For this review, take the finished solid that the model builds, in its own axes (mm). Face numbers are marked on the shaded views. Coordinates: 2 decimals unless noted, no trailing zeros. Order: outer loops, then holes, each group sorted by start corner. A loop starts at its lowest first (then second) coordinate and runs counter-clockwise, first axis right, second up. Notation, with made-up numbers: M 72,27 L 128,27 A29 ccw 128,61 Z; hole C 68.25,-2 d5. An arc over 180 degrees is marked long. Use CSV: the item, a comma, the result in double quotes.
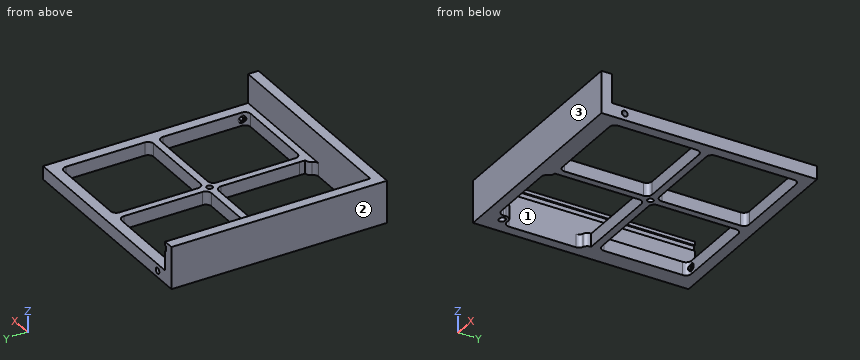
```python
from build123d import *

# Parameters (mm, degrees)
BOSS_EXTRUDE1_DEPTH            = 23
SKETCH2_W                      = 3
SKETCH2_H                      = 112
CUT_EXTRUDE1_DEPTH             = 0.75
SKETCH3_W                      = 7.2
SKETCH3_H                      = 6
BOSS_EXTRUDE2_DEPTH            = 10
SKETCH3_3_W                    = 7.2
SKETCH3_3_H                    = 106
BOSS_EXTRUDE3_DEPTH            = 4
FILLET1_R                      = 3
SKETCH5_W                      = 101.3
SKETCH5_H                      = 7.2
BOSS_EXTRUDE4_DEPTH            = 4
SKETCH5_3_W                    = 6
SKETCH5_3_H                    = 7.2
BOSS_EXTRUDE5_DEPTH            = 10
FILLET3_R                      = 3
SKETCH6_W                      = 50
SKETCH6_H                      = 50
CUT_EXTRUDE2_DEPTH             = 167.709117927
FILLET8_R                      = 3
FILLET9_R                      = 3
FILLET10_R                     = 3
FILLET11_R                     = 3
CUT_EXTRUDE3_REACH             = 169.545
SKETCH7_R                      = 1
CUT_EXTRUDE3_DIRECTION_2_DEPTH = 168.544889647
SKETCH7_5_R                    = 1.6
SKETCH7_5_R_2                  = 1
CUT_EXTRUDE4_DEPTH             = 3.2
CUT_EXTRUDE6_START             = -5.5
SKETCH8_R                      = 2
CUT_EXTRUDE6_DEPTH             = 3
CUT_EXTRUDE7_REACH             = 169.545
SKETCH9_R                      = 1
SKETCH9_3_R                    = 1.6
SKETCH9_3_R_2                  = 1
CUT_EXTRUDE8_DEPTH             = 3.2
CUT_EXTRUDE9_START             = -5.5
SKETCH10_R                     = 2
CUT_EXTRUDE9_DEPTH             = 3.2
BOSS_EXTRUDE6_DEPTH            = 7.2
FILLET12_R                     = 3
BOSS_EXTRUDE7_DEPTH            = 7.2
FILLET13_R                     = 3
FILLET14_R                     = 3
FILLET15_R                     = 3
FILLET16_R                     = 3
BOSS_EXTRUDE8_DEPTH            = 7.2
CUT_EXTRUDE10_REACH            = 168.709
CUT_EXTRUDE11_DEPTH            = 7.2
FILLET17_R                     = 3
CUT_EXTRUDE12_REACH            = 169.545
SKETCH16_R                     = 1.6


with BuildPart() as part:
    # Sketch1 → Boss-Extrude1 (new body)
    with BuildSketch(Plane.XY):
        Polygon((0, 117.7), (0, 0), (117, 0), (117, 5.7), (5.7, 5.7), (5.7, 117.7), align=None)
    extrude(amount=BOSS_EXTRUDE1_DEPTH)

    # Sketch2 → Cut-Extrude1 (cut)
    with BuildSketch(Plane(origin=(5.7, 0, 0), x_dir=(0, 0, -1), z_dir=(1, 0, 0))):
        with Locations((-19.5, 61.7)):
            Rectangle(SKETCH2_W, SKETCH2_H)
    extrude(amount=-CUT_EXTRUDE1_DEPTH, mode=Mode.SUBTRACT)

    # Sketch3 → Boss-Extrude2 (add)
    with BuildSketch(Plane(origin=(5.7, 0, 0), x_dir=(0, 0, -1), z_dir=(1, 0, 0))):
        with Locations((-3.6, 114.7)):
            Rectangle(SKETCH3_W, SKETCH3_H)
    extrude(amount=BOSS_EXTRUDE2_DEPTH)

    # Sketch3<3> → Boss-Extrude3 (add)
    with BuildSketch(Plane(origin=(5.7, 0, 0), x_dir=(0, 0, -1), z_dir=(1, 0, 0))):
        with Locations((-3.6, 58.7)):
            Rectangle(SKETCH3_3_W, SKETCH3_3_H)
    extrude(amount=BOSS_EXTRUDE3_DEPTH)

    # Fillet1
    fillet1_edges = [part.edges().sort_by_distance(p)[0] for p in [
        (9.7, 111.7, 3.6),
    ]]
    fillet(fillet1_edges, radius=FILLET1_R)

    # Sketch5 → Boss-Extrude4 (add)
    with BuildSketch(Plane(origin=(0, 5.7, 0), x_dir=(1, 0, 0), z_dir=(0, 1, 0))):
        with Locations((60.35, -3.6)):
            Rectangle(SKETCH5_W, SKETCH5_H)
    extrude(amount=BOSS_EXTRUDE4_DEPTH)

    # Sketch5<3> → Boss-Extrude5 (add)
    with BuildSketch(Plane(origin=(0, 5.7, 0), x_dir=(1, 0, 0), z_dir=(0, 1, 0))):
        with Locations((114, -3.6)):
            Rectangle(SKETCH5_3_W, SKETCH5_3_H)
    extrude(amount=BOSS_EXTRUDE5_DEPTH)

    # Fillet3
    fillet3_edges = [part.edges().sort_by_distance(p)[0] for p in [
        (111, 9.7, 3.6),
    ]]
    fillet(fillet3_edges, radius=FILLET3_R)

    # Sketch6 → Cut-Extrude2 (cut, through all)
    with BuildSketch(Plane.XY.offset(7.2)):
        with Locations((30.7, 30.7)):
            Rectangle(SKETCH6_W, SKETCH6_H)
    extrude(amount=-CUT_EXTRUDE2_DEPTH, mode=Mode.SUBTRACT)

    # Fillet8
    fillet8_edges = [part.edges().sort_by_distance(p)[0] for p in [
        (5.7, 55.7, 3.6),
    ]]
    fillet(fillet8_edges, radius=FILLET8_R)

    # Fillet9
    fillet9_edges = [part.edges().sort_by_distance(p)[0] for p in [
        (9.7, 55.7, 3.6),
    ]]
    fillet(fillet9_edges, radius=FILLET9_R)

    # Fillet10
    fillet10_edges = [part.edges().sort_by_distance(p)[0] for p in [
        (55.7, 5.7, 3.6),
    ]]
    fillet(fillet10_edges, radius=FILLET10_R)

    # Fillet11
    fillet11_edges = [part.edges().sort_by_distance(p)[0] for p in [
        (55.7, 9.7, 3.6),
    ]]
    fillet(fillet11_edges, radius=FILLET11_R)

    # Sketch7 → Cut-Extrude3 (cut, up to next)
    with BuildSketch(Plane(origin=(117, 0, 0), x_dir=(0, 0, -1), z_dir=(1, 0, 0)), mode=Mode.PRIVATE) as cut_extrude3_sk1:
        with Locations(Location((-3.6, 12.7, 0), (0, 0, 180))):
            Circle(SKETCH7_R)
    cut_extrude3_tool1 = extrude(cut_extrude3_sk1.sketch, amount=-CUT_EXTRUDE3_REACH, mode=Mode.PRIVATE) & part.part
    add(cut_extrude3_tool1.solids().sort_by_distance((117, 12.7, 3.6))[0], mode=Mode.SUBTRACT)

    # Sketch7 → Cut-Extrude3 direction 2 (cut)
    with BuildSketch(Plane(origin=(117, 0, 0), x_dir=(0, 0, -1), z_dir=(1, 0, 0))):
        with Locations(Location((-3.6, 12.7, 0), (0, 0, 180))):
            Circle(SKETCH7_R)
    extrude(amount=CUT_EXTRUDE3_DIRECTION_2_DEPTH, mode=Mode.SUBTRACT)

    # Sketch7<5> → Cut-Extrude4 (cut)
    with BuildSketch(Plane(origin=(117, 0, 0), x_dir=(0, 0, -1), z_dir=(1, 0, 0))):
        with Locations((-3.6, 12.7)):
            Circle(SKETCH7_5_R)
        with Locations((-3.6, 12.7)):
            Circle(SKETCH7_5_R_2, mode=Mode.SUBTRACT)
    extrude(amount=-CUT_EXTRUDE4_DEPTH, mode=Mode.SUBTRACT)

    # Sketch8 → Cut-Extrude6 (cut)
    with BuildSketch(Plane(origin=(117, 0, 0), x_dir=(0, 0, -1), z_dir=(1, 0, 0)).offset(CUT_EXTRUDE6_START)):
        with Locations((-3.6, 12.7)):
            Circle(SKETCH8_R)
    extrude(amount=-CUT_EXTRUDE6_DEPTH, mode=Mode.SUBTRACT)

    # Sketch9 → Cut-Extrude7 (cut, up to next)
    with BuildSketch(Plane(origin=(0, 117.7, 0), x_dir=(1, 0, 0), z_dir=(0, 1, 0)), mode=Mode.PRIVATE) as cut_extrude7_sk1:
        with Locations(Location((12.7, -3.6, 0), (0, 0, 270))):
            Circle(SKETCH9_R)
    cut_extrude7_tool1 = extrude(cut_extrude7_sk1.sketch, amount=-CUT_EXTRUDE7_REACH, mode=Mode.PRIVATE) & part.part
    add(cut_extrude7_tool1.solids().sort_by_distance((12.7, 117.7, 3.6))[0], mode=Mode.SUBTRACT)

    # Sketch9<3> → Cut-Extrude8 (cut)
    with BuildSketch(Plane(origin=(0, 117.7, 0), x_dir=(1, 0, 0), z_dir=(0, 1, 0))):
        with Locations(Location((12.7, -3.6, 0), (0, 0, 270))):
            Circle(SKETCH9_3_R)
        with Locations(Location((12.7, -3.6, 0), (0, 0, 270))):
            Circle(SKETCH9_3_R_2, mode=Mode.SUBTRACT)
    extrude(amount=-CUT_EXTRUDE8_DEPTH, mode=Mode.SUBTRACT)

    # Sketch10 → Cut-Extrude9 (cut)
    with BuildSketch(Plane(origin=(0, 117.7, 0), x_dir=(1, 0, 0), z_dir=(0, 1, 0)).offset(CUT_EXTRUDE9_START)):
        with Locations(Location((12.7, -3.6, 0), (0, 0, 270))):
            Circle(SKETCH10_R)
    extrude(amount=-CUT_EXTRUDE9_DEPTH, mode=Mode.SUBTRACT)

    # Sketch11 → Boss-Extrude6 (add)
    with BuildSketch(Plane(origin=(0, 0, 0), x_dir=(-1, 0, 0), z_dir=(0, 0, -1))):
        Polygon((-117, 15.7), (-111, 15.7), (-111, 111.7), (-15.7, 111.7), (-15.7, 117.7), (-63.35, 117.7), (-117, 117.7), align=None)
    extrude(amount=-BOSS_EXTRUDE6_DEPTH)

    # Fillet12
    fillet12_edges = [part.edges().sort_by_distance(p)[0] for p in [
        (111, 111.7, 3.6),
    ]]
    fillet(fillet12_edges, radius=FILLET12_R)

    # Sketch12 → Boss-Extrude7 (add)
    with BuildSketch(Plane(origin=(0, 0, 0), x_dir=(-1, 0, 0), z_dir=(0, 0, -1))):
        Polygon((-62.35, 12.7), (-62.35, 9.7), (-58.356854249, 9.7), (-58.35, 12.7), (-58.35, 58.7), (-9.7, 58.7), (-9.7, 62.7), (-58.35, 62.7), (-58.35, 108.7), (-58.35, 111.7), (-62.35, 111.7), (-62.35, 108.7), (-62.35, 62.7), (-111, 62.7), (-111, 58.7), (-62.35, 58.7), align=None)
    extrude(amount=-BOSS_EXTRUDE7_DEPTH)

    # Fillet13
    fillet13_edges = [part.edges().sort_by_distance(p)[0] for p in [
        (111, 62.7, 3.6),
        (62.35, 62.7, 3.6),
        (62.35, 111.7, 3.6),
    ]]
    fillet(fillet13_edges, radius=FILLET13_R)

    # Fillet14
    fillet14_edges = [part.edges().sort_by_distance(p)[0] for p in [
        (111, 58.7, 3.6),
        (62.35, 9.7, 3.6),
        (62.35, 58.7, 3.6),
    ]]
    fillet(fillet14_edges, radius=FILLET14_R)

    # Fillet15
    fillet15_edges = [part.edges().sort_by_distance(p)[0] for p in [
        (58.35, 111.7, 3.6),
        (58.35, 62.7, 3.6),
        (9.7, 62.7, 3.6),
    ]]
    fillet(fillet15_edges, radius=FILLET15_R)

    # Fillet16
    fillet16_edges = [part.edges().sort_by_distance(p)[0] for p in [
        (58.35, 58.7, 3.6),
    ]]
    fillet(fillet16_edges, radius=FILLET16_R)

    # Sketch13 → Boss-Extrude8 (add)
    with BuildSketch(Plane(origin=(0, 0, 0), x_dir=(-1, 0, 0), z_dir=(0, 0, -1))):
        Polygon((-5.7, 20.7), (-20.7, 5.7), (-5.7, 5.7), align=None)
    extrude(amount=-BOSS_EXTRUDE8_DEPTH)

    # Sketch14 → Cut-Extrude10 (cut, up to next)
    with BuildSketch(Plane.XY.offset(7.2), mode=Mode.PRIVATE) as cut_extrude10_sk1:
        with BuildLine():
            Line((10, 8.6), (9.2, 8.6))
            ThreePointArc((9.2, 8.6), (7.6, 10.2), (9.2, 11.8))
            Line((9.2, 11.8), (10, 11.8))
            ThreePointArc((10, 11.8), (11.6, 10.2), (10, 8.6))
        make_face()
    cut_extrude10_tool1 = extrude(cut_extrude10_sk1.sketch, amount=-CUT_EXTRUDE10_REACH, mode=Mode.PRIVATE) & part.part
    add(cut_extrude10_tool1.solids().sort_by_distance((9.6, 10.2, 7.2))[0], mode=Mode.SUBTRACT)

    # Sketch15 → Cut-Extrude11 (cut)
    with BuildSketch(Plane.XY.offset(7.2)):
        Polygon((13.2, 5.7), (20.7, 5.7), (13.2, 13.2), align=None)
        Polygon((5.7, 13.2), (13.2, 13.2), (5.7, 20.7), align=None)
        Polygon((13.2, 13.2), (20.7, 5.7), (20.7, 13.2), (20.7, 20.7), (13.2, 20.7), (5.7, 20.7), align=None)
    extrude(amount=-CUT_EXTRUDE11_DEPTH, mode=Mode.SUBTRACT)

    # Fillet17
    fillet17_edges = [part.edges().sort_by_distance(p)[0] for p in [
        (5.7, 13.2, 3.6),
        (13.2, 5.7, 3.6),
        (13.2, 13.2, 3.6),
    ]]
    fillet(fillet17_edges, radius=FILLET17_R)

    # Sketch16 → Cut-Extrude12 (cut, up to next)
    with BuildSketch(Plane(origin=(0, 0, 0), x_dir=(-1, 0, 0), z_dir=(0, 0, -1)), mode=Mode.PRIVATE) as cut_extrude12_sk1:
        with Locations((-60.35, 60.7)):
            Circle(SKETCH16_R)
    cut_extrude12_tool1 = extrude(cut_extrude12_sk1.sketch, amount=-CUT_EXTRUDE12_REACH, mode=Mode.PRIVATE) & part.part
    add(cut_extrude12_tool1.solids().sort_by_distance((60.35, 60.7, 0))[0], mode=Mode.SUBTRACT)


solid = part.part
```
Item 1: Add section D-D on z = 9.5. State the section outline as (x, y) points, and give its area (3 significant figures).
Solutions:
outline,"M 0,0 L 117,0 L 117,5.7 L 5.7,5.7 L 5.7,117.7 L 0,117.7 Z"
area,"1,310 mm^2"
Item 2: Clearance check with flat-ended pins moving along their axes: pin 1 Ø3.5 at (y, z) = (35, 19.5) entering from +X; pin 2 Ø2.5 at (y, z) = (12.7, 3.6) entering from +X; pin 3 Ø1.5 at (x, z) = (37.5, 14) entering from +Y. State where each tip first meets the part, or that it passes through.
Solutions:
pin 1,"x = 5.7"
pin 2,"x = 113.8"
pin 3,"y = 5.7"
Item 3: Add section C-C on y = 60.7. State the section outline as (x, z) points.
Solutions:
outline,"M 0,0 L 58.75,0 L 58.75,7.2 L 5.7,7.2 L 5.7,18 L 4.95,18 L 4.95,21 L 5.7,21 L 5.7,23 L 0,23 Z; M 61.95,0 L 117,0 L 117,7.2 L 61.95,7.2 Z"
Item 4: Add section B-B on y = 93.5. State the section outline as (x, z) points, and give its area (3 significant figures).
Solutions:
outline,"M 0,0 L 9.7,0 L 9.7,7.2 L 5.7,7.2 L 5.7,18 L 4.95,18 L 4.95,21 L 5.7,21 L 5.7,23 L 0,23 Z; M 58.35,0 L 62.35,0 L 62.35,7.2 L 58.35,7.2 Z; M 111,0 L 117,0 L 117,7.2 L 111,7.2 Z"
area,"230 mm^2"
Item 5: Draft analysis for pull direction X (two halves, no side actions). For the marked faces 1, 2 and 3, state which applies: released by +X, released by -X, zero draft, split by the parting line, or undercut.
Solutions:
face 1,"undercut"
face 2,"released by -X"
face 3,"zero draft"
Item 6: To check wall thickness, follow line 1 along X through (y, z) = (111.85, 3.6); line 2 along Y through (x, z) = (115.6, 3.6); line 3 along Y through (x, z) = (100.5, 1.5). State the ranges of each line that lie inside material, in increasing order. Write a range as [from, to].
Solutions:
line 1,"[0, 10.7], [14.7, 117]"
line 2,"[0, 11.1], [14.3, 117.7]"
line 3,"[0, 9.7], [58.7, 62.7], [111.7, 117.7]"
Item 7: Add section A-A on x = 20. State the section outline as (y, z) points.
Solutions:
outline,"M 0,0 L 5.7,0 L 5.7,23 L 0,23 Z; M 58.7,0 L 62.7,0 L 62.7,7.2 L 58.7,7.2 Z; M 111.7,0 L 117.7,0 L 117.7,7.2 L 111.7,7.2 Z"
